Model file for the job. Use its own axes, mm. Face numbers are marked on the shaded views. A direction names the side the tool comes from. Coordinates: 2 decimals unless noted, no trailing zeros. Order: outer loops, then holes, each group sorted by start corner. A loop starts at its lowest first (then second) coordinate and runs counter-clockwise, first axis right, second up. Notation, with made-up numbers: (38, 16) -> (57, 16) arc R19 ccw to (57, 33) -> close; hole circle Ø5 at (-15.5, 44). An arc over 180 degrees is marked (long way). Write item = value, one per line. Start each with the question number.
Q1. Wall check: line 1 (Z direction, x = 38, y = -11) (3 decimals); line 2 (Z direction, x = 16, y = 33) (3 decimals); line 3 (X direction, y = 16, z = 368). Give the ranges that are in metal, low to high. Write a range as from..to.
Q2. Flat gauge pins, fed straight in: pin 1 (1.5 mm diameter, centred on x = -21.5, y = 41.5, fed in from +Z); pin 2 (1.5 mm diameter, centred on x = -52.5, z = -324, fed in from +Y). Where does each tip first touch, or does it go through?
Q3. Cut at D-D, the plane x = -65. List the corners of the cut face in (y, z) (3 decimals).
Q4. 3-axis set-ups, long thin cutter, end or side, ignore diameter. For the marked faces 3 and 4: which of +Z, -Z, +X, -X, +Y, -Y reach the whole face in a straight line?
Q5. Cut at A-A, the plane x = 34. List the corners of the cut face in (y, z) (3 decimals), plus the area to 3 significant figures.
Q6. Mould opens along Z. For the marked faces 1 and 2 say: +Z half, -Z half, draft (parallel to the pull), parting line (faces both ways), or undercut.
Q7. Cut at C-C, the plane z = 255. List the corners of the cut face in (x, y).
Q8. Cut at B-B, the plane y = -46. List the corners of the cut face in (x, z) (3 decimals).
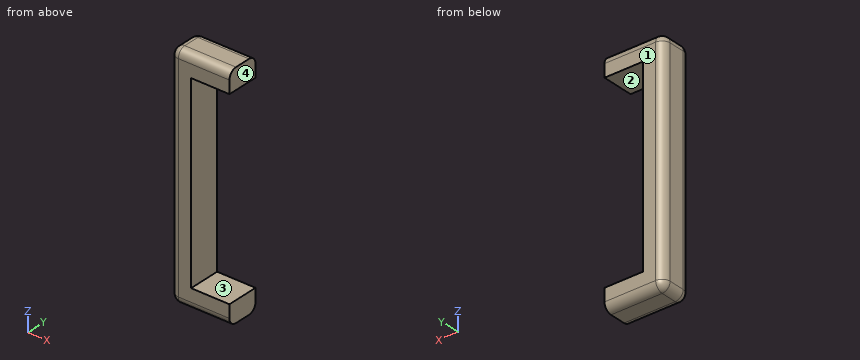
from build123d import *

# Parameters (mm, degrees)
BOSS_EXTRUDE1_DEPTH = 63.5
FILLET1_R           = 31.75


with BuildPart() as part:
    # Sketch1 → Boss-Extrude1 (new body, symmetric)
    with BuildSketch(Plane(origin=(0, 0, 0), x_dir=(1, 0, 0), z_dir=(0, 1, 0))):
        with BuildLine():
            Line((0, 377.825), (0, -377.825))
            Line((0, -377.825), (152.4, -377.825))
            Line((152.4, -377.825), (152.4, -460.375))
            Line((152.4, -460.375), (-50.8, -460.375))
            ThreePointArc((-50.8, -460.375), (-73.250640303, -451.075640303), (-82.55, -428.625))
            Line((-82.55, -428.625), (-82.55, 428.625))
            ThreePointArc((-82.55, 428.625), (-73.250640303, 451.075640303), (-50.8, 460.375))
            Line((-50.8, 460.375), (152.4, 460.375))
            Line((152.4, 460.375), (152.4, 377.825))
            Line((152.4, 377.825), (0, 377.825))
        make_face()
    extrude(amount=BOSS_EXTRUDE1_DEPTH, both=True)

    # Fillet1
    fillet1_edges = [part.edges().sort_by_distance(p)[0] for p in [
        (-73.250640303, -63.5, 451.075640303),
        (-82.55, -63.5, 0),
        (-73.250640303, -63.5, -451.075640303),
        (50.8, -63.5, -460.375),
        (50.8, 63.5, -460.375),
        (-73.250640303, 63.5, -451.075640303),
        (-82.55, 63.5, 0),
        (-73.250640303, 63.5, 451.075640303),
        (50.8, 63.5, 460.375),
        (50.8, -63.5, 460.375),
    ]]
    fillet(fillet1_edges, radius=FILLET1_R)


solid = part.part
Here are the results:
q1.line_1 = -460.375..-377.825, 377.825..460.375
q1.line_2 = -460.35..-377.825, 377.825..460.35
q1.line_3 = -82.55..0
q2.pin_1 = 459.07
q2.pin_2 = 63.49
q3.outline = (-60.148, -428.625) arc R28.398 ccw to (-31.75, -457.023) -> (31.75, -457.023) arc R28.398 ccw to (60.148, -428.625) -> (60.148, 428.625) arc R28.398 ccw to (31.75, 457.023) -> (-31.75, 457.023) arc R28.398 ccw to (-60.148, 428.625) -> close
q4.face_3 = +X, +Y, -Y
q4.face_4 = +Z, -Z, +X, +Y, -Y
q5.outline = (-63.5, -428.625) arc R31.75 ccw to (-31.75, -460.375) -> (31.75, -460.375) arc R31.75 ccw to (63.5, -428.625) -> (63.5, -377.825) -> (-63.5, -377.825) -> close; (-63.5, 377.825) -> (63.5, 377.825) -> (63.5, 428.625) arc R31.75 ccw to (31.75, 460.375) -> (-31.75, 460.375) arc R31.75 ccw to (-63.5, 428.625) -> close
q5.area = 20,100 mm²
q6.face_1 = draft
q6.face_2 = undercut
q7.outline = (-82.55, -31.75) arc R31.75 ccw to (-50.8, -63.5) -> (0, -63.5) -> (0, 63.5) -> (-50.8, 63.5) arc R31.75 ccw to (-82.55, 31.75) -> close
q8.outline = (-79.173, -428.625) arc R28.373 ccw to (-50.8, -456.998) -> (152.4, -456.998) -> (152.4, -377.825) -> (0, -377.825) -> (0, 377.825) -> (152.4, 377.825) -> (152.4, 456.998) -> (-50.8, 456.998) arc R28.373 ccw to (-79.173, 428.625) -> close
